Verification items for the finished model (mm, model axes). A direction names the side the tool comes from. Give positions to 0.01 mm unless a question says otherwise; leave off trailing zeros. Loops run counter-clockwise (first coordinate to the right, second up) from the corner with the lowest first, then second, coordinate; pieces in that order, holes last. Notation, with made-up numbers: (78.5, 0.25) - (132.5, 0.25) arc R13 cw to (132.5, 15.25) - close; hole circle Ø1 at (-4, 21.5). An arc over 180 degrees is marked (long way). One line per item, written item: value. Start each with the question number.
1. Sectioned sample at D-D (y = 53.5). Record the cut outline in (x, z) (3 decimals).
2. Sectioned sample at A-A (z = 3). Record the cut outline in (x, y), plus the area to 3 significant figures.
3. Access from +Z, -Z, +X, -X, +Y, -Y to the whole of each face (thin tool, end or side, straight path). Record for faces 1 (the flat face through (-1, 89.687, 6)), 2 (the flat face through (40.365, 71, 6)), 3 (the flat face through (-1, 55.096, 5)), 4 (the flat face through (-40.365, 71, 6)), 5 (the flat face through (-1, 52.517, 6)).
4. Mould release check, pull along Y, two halves, no side actions. Record for faces 6 (the flat face through (-43, 71, 2)), 7 (the flat face through (-1, 92.103, 2)), 8 (the flat face through (-1, 87.096, 5)): pulls with the +Y half, pulls with the -Y half, needs draft (parallel to the pull), parting line crosses it, or undercut.
5. Scan lines: L1, parallel to Y at x = 25.5, z = 3; L2, parallel to Y at x = -19.5, z = 6.25; L3, parallel to X at y = 57, z = 4.5. Record each from-to range of solid material in increasing order. Write a range as [from, to].
6. Sectioned sample at B-B (y = 59). Record the cut outline in (x, z) (3 decimals), plus the area to 3 significant figures.
7. Sectioned sample at C-C (x = 35). Record the cut outline in (y, z), plus the area to 3 significant figures.
8. Gauge pin test, flat ends, axial feed: pin 1 (2 mm diameter, centred on x = 1.5, z = 6.5, fed in from -Y); pin 2 (1 mm diameter, centred on y = 75.5, z = 6, fed in from -X) (3 decimals); pin 3 (1.6 mm diameter, centred on y = 70.5, z = 6, fed in from +X) (3 decimals); pin 4 (12 mm diameter, centred on x = 5.5, y = 60.5, fed in from -Z). Record the tip position at first contact, or that the pin passes through.
from build123d import *

# Parameters (mm, degrees)
SKETCH010_W     = 86
SKETCH010_H     = 42
PAD004_DEPTH    = 5
SKETCH012_W     = 80.73
SKETCH012_H     = 37.17
PAD005_DEPTH    = 2
SKETCH013_W     = 78
SKETCH013_H     = 32
POCKET006_DEPTH = 5


with BuildPart() as part:
    # Sketch010 → Pad004 (new body)
    with BuildSketch(Plane.XY):
        with Locations((0, 71.102745)):
            Rectangle(SKETCH010_W, SKETCH010_H)
    extrude(amount=PAD004_DEPTH)

    # Sketch012 (on Face6 of Pad004) → Pad005 (join)
    with BuildSketch(Plane.XY.offset(5)):
        with Locations((0, 71.102234)):
            Rectangle(SKETCH012_W, SKETCH012_H)
    extrude(amount=PAD005_DEPTH)

    # Sketch013 (on Face11 of Pad005) → Pocket006 (cut)
    with BuildSketch(Plane.XY.offset(7)):
        with Locations((0, 71.096275)):
            Rectangle(SKETCH013_W, SKETCH013_H)
    extrude(amount=-POCKET006_DEPTH, mode=Mode.SUBTRACT)


solid = part.part
Results are:
1. outline: (-43, 0) - (43, 0) - (43, 5) - (40.365, 5) - (40.365, 7) - (-40.365, 7) - (-40.365, 5) - (-43, 5) - close
2. outline: (-43, 50.1) - (43, 50.1) - (43, 92.1) - (-43, 92.1) - close; hole (-39, 55.1) - (39, 55.1) - (39, 87.1) - (-39, 87.1) - close
2. area: 1,120 mm^2
3. face 1: +Z, +X, -X, +Y
3. face 2: +Z, +X, +Y, -Y
3. face 3: +Z
3. face 4: +Z, -X, +Y, -Y
3. face 5: +Z, +X, -X, -Y
4. face 6: needs draft
4. face 7: pulls with the +Y half
4. face 8: undercut
5. L1: y = [50.1, 55.1], [87.1, 92.1]
5. L2: y = [52.52, 55.1], [87.1, 89.69]
5. L3: x = [-43, -39], [39, 43]
6. outline: (-43, 0) - (43, 0) - (43, 5) - (40.365, 5) - (40.365, 7) - (39, 7) - (39, 2) - (-39, 2) - (-39, 7) - (-40.365, 7) - (-40.365, 5) - (-43, 5) - close
6. area: 201 mm^2
7. outline: (50.1, 0) - (92.1, 0) - (92.1, 5) - (89.69, 5) - (89.69, 7) - (87.1, 7) - (87.1, 2) - (55.1, 2) - (55.1, 7) - (52.52, 7) - (52.52, 5) - (50.1, 5) - close
7. area: 124 mm^2
8. pin 1: stops at y = 52.52
8. pin 2: stops at x = -40.365
8. pin 3: stops at x = 40.365
8. pin 4: stops at z = 0
